Autodesk Inventor part; units mm, degrees
ref_plane "YZ Plane" through (0, 0, 0) normal (1, 0, 0) x (0, 1, 0)
ref_plane "XZ Plane" through (0, 0, 0) normal (0, 1, 0) x (-1, 0, 0)
ref_plane "XY Plane" through (0, 0, 0) normal (0, 0, 1) x (1, 0, 0)
sketch "Sketch1" plane through (0, 0, 0) normal (0, 1, 0) x (-1, 0, 0)
  line L0 (0, 0) -> (25.5, 0)
  line L1 (25.5, 0) -> (25.5, -75.4)
  line L2 (25.5, -75.4) -> (0, -75.4)
  line L3 (0, -75.4) -> (0, 0)
  dimension "d0" = 25.5
  dimension "d1" = 75.4
extrude "Extrusion1" add sketch "Sketch1" along normal blind 1.6
sketch "Sketch2" plane through (0, 1.6, 0) normal (0, 1, 0) x (1, 0, 0)
  line L0 (-25.5, 0) -> (0, 0)
  line L1 (0, 0) -> (0, 75.4)
  line L2 (0, 75.4) -> (-25.5, 75.4)
  line L3 (-25.5, 75.4) -> (-25.5, 0)
  circle A0 centre (-22.5, 71.4) radius 1.75
  circle A1 centre (-22.5, 62.9) radius 1.75
  circle A2 centre (-22.5, 53.4) radius 1.75
  circle A3 centre (-22.5, 48.9) radius 1.75
  line L4 (-25.5, 0) -> (0, 0) construction
  line L5 (-12.75, 0) -> (-12.75, 75.4) construction
  line L6 (0, 75.4) -> (-25.5, 75.4) construction
  line L7 (-25.5, 75.4) -> (-25.5, 0) construction
  line L8 (-25.5, 37.7) -> (0, 37.7) construction
  circle A4 centre (-3, 71.4) radius 1.75
  circle A5 centre (-3, 62.9) radius 1.75
  circle A6 centre (-3, 53.4) radius 1.75
  circle A7 centre (-3, 48.9) radius 1.75
  circle A8 centre (-22.5, 4) radius 1.75
  circle A9 centre (-22.5, 12.5) radius 1.75
  circle A10 centre (-22.5, 22) radius 1.75
  circle A11 centre (-22.5, 26.5) radius 1.75
  circle A12 centre (-3, 22) radius 1.75
  circle A13 centre (-3, 12.5) radius 1.75
  circle A14 centre (-3, 4) radius 1.75
  circle A15 centre (-3, 26.5) radius 1.75
  dimension "d4" = 3.5
  dimension "d5" = 3
  dimension "d6" = 4
  dimension "d7" = 3.5
  dimension "d8" = 12.5
  dimension "d9" = 3.5
  dimension "d10" = 22
  dimension "d11" = 3.5
  dimension "d12" = 26.5
extrude "Extrusion2" add sketch "Sketch2" along normal blind 3 contours A0 | A1 | A2 | A3 | A4 | A5 | A6 | A7 | A8 | A9 | A10 | A11 | A12 | A13 | A14 | A15
sketch "Sketch3" plane through (0, 1.6, 0) normal (0, 1, 0) x (1, 0, 0)
  circle A0 centre (-22.5, 4) radius 1.75
  circle A1 centre (-22.5, 12.5) radius 1.75
  circle A2 centre (-22.5, 22) radius 1.75
  circle A3 centre (-22.5, 26.5) radius 1.75
  circle A4 centre (-3, 71.4) radius 1.75
  circle A5 centre (-3, 53.4) radius 1.75
  circle A6 centre (-22.5, 53.4) radius 1.75
  circle A7 centre (-22.5, 71.4) radius 1.75
  circle A8 centre (-22.5, 62.9) radius 1.75
  circle A9 centre (-22.5, 48.9) radius 1.75
  circle A10 centre (-3, 62.9) radius 1.75
  circle A11 centre (-3, 48.9) radius 1.75
  circle A12 centre (-3, 26.5) radius 1.75
  circle A13 centre (-3, 22) radius 1.75
  circle A14 centre (-3, 12.5) radius 1.75
  circle A15 centre (-3, 4) radius 1.75
  line L0 (-25.5, 0) -> (0, 0)
  line L1 (0, 0) -> (0, 75.4)
  line L2 (0, 75.4) -> (-25.5, 75.4)
  line L3 (-25.5, 75.4) -> (-25.5, 0)
  line L4 (-16.8, 61.4) -> (-9.8, 61.4)
  line L5 (-9.8, 61.4) -> (-9.8, 50.4)
  line L6 (-9.8, 50.4) -> (-16.8, 50.4)
  line L7 (-16.8, 50.4) -> (-16.8, 61.4)
  line L8 (-25.5, 0) -> (-25.5, 75.4)
  line L9 (-25.5, 37.7) -> (0, 37.7)
  line L10 (0, 75.4) -> (0, 0)
  line L11 (-16.8, 14) -> (-9.8, 14)
  line L12 (-9.8, 14) -> (-9.8, 25)
  line L13 (-9.8, 25) -> (-16.8, 25)
  line L14 (-16.8, 25) -> (-16.8, 14)
  circle A16 centre (-13.3, 55.9) radius 4.511
  circle A17 centre (-13.3, 19.5) radius 4.5729
  dimension "d15" = 7
  dimension "d16" = 11
  dimension "d17" = 14
  dimension "d18" = 8.7
extrude "Extrusion3" cut sketch "Sketch3" against normal blind 3 contours L4 L5 A16 L7 | A16 L5 L7 | L7 A16 | A16 L5 | A16 L5 L6 L7 | L14 A17 L12 L11 | A17 L14 | L14 A17 L12 | L12 A17 | L14 L13 L12 A17
properties part number "00_FluidicChip_AlexSwen"
The model under review builds one solid part; all positions refer to its coordinate system, in mm. A direction names the side the tool comes from. Give positions to 0.01 mm unless a question says otherwise; leave off trailing zeros. Write each loop counter-clockwise with the first axis right and the second up, starting at its lowest first coordinate (ties: lowest second). Pieces come first, ordered by that corner, then holes. Notation, with made-up numbers: M -7,88.25 L 2,88.25 A36 ccw 2,122.25 Z; hole C -30.75,45.5 d9. An arc over 180 degrees is marked long. One line per question, with ' | ' between items. Start each with the question number.
Item 1: We need section A-A on y = 3.4. Give the number of separate pieces and of enclosed holes in the cut face, plus the area to 3 significant figures.
Item 2: We need section C-C on z = -12.5. Write out the cut boundary in (x, y).
Item 3: We need section D-D on x = -18.75. Write out the cut boundary in (y, z).
Item 4: Draft analysis for pull direction Z (two halves, no side actions). For faces 1 (the cylindrical face through (-3.228, 3.079, -61.165)), 2 (the flat face through (-3, 4.6, -63)), state which applies: released by +Z, released by -Z, zero draft, split by the parting line, or undercut.
Item 5: We need section B-B on x = -13.5. Write out the cut boundary in (y, z), plus the area to 3 significant figures.
Item 6: Wall thickness on line 1 (Z direction, x = -10.75, y = 1.4); line 2 (X direction, y = 3.1, z = -22); line 3 (X direction, y = 0.7, z = -61): over which ranges is each line inside the solid? List them lowest first. Write a range as from..to.
Item 7: For faces 3 (the cylindrical face through (-17.873, 0.811, -19.545)), 4 (the flat face through (-23, 4.6, -49)), 5 (the cylindrical face through (-22.728, 3.079, -61.165)), list the 3-axis set-ups (+Z, -Z, +X, -X, +Y, -Y) from which the entire face can be reached by the end or side of a thin tool; tool diameter is ignored.
Results found:
1) separate pieces: 16 | enclosed holes: 0 | area: 154 mm2
2) outline: M -25.5,0 L 0,0 L 0,1.6 L -1.25,1.6 L -1.25,4.6 L -4.75,4.6 L -4.75,1.6 L -20.75,1.6 L -20.75,4.6 L -24.25,4.6 L -24.25,1.6 L -25.5,1.6 Z
3) outline: M 0,-75.4 L 1.6,-75.4 L 1.6,0 L 0,0 Z
4) face 1: undercut | face 2: zero draft
5) outline: M 0,-75.4 L 1.6,-75.4 L 1.6,-61.4 L 0,-61.4 Z; M 0,-50.4 L 1.6,-50.4 L 1.6,-25 L 0,-25 Z; M 0,-14 L 1.6,-14 L 1.6,0 L 0,0 Z | area: 85.4 mm2
6) line 1: z = -75.4..-61.4, -50.4..-25, -14..0 | line 2: x = -24.25..-20.75, -4.75..-1.25 | line 3: x = -25.5..-16.8, -9.8..0
7) face 3: +Y, -Y | face 4: +Z, -Z, +X, -X, +Y | face 5: +Y
